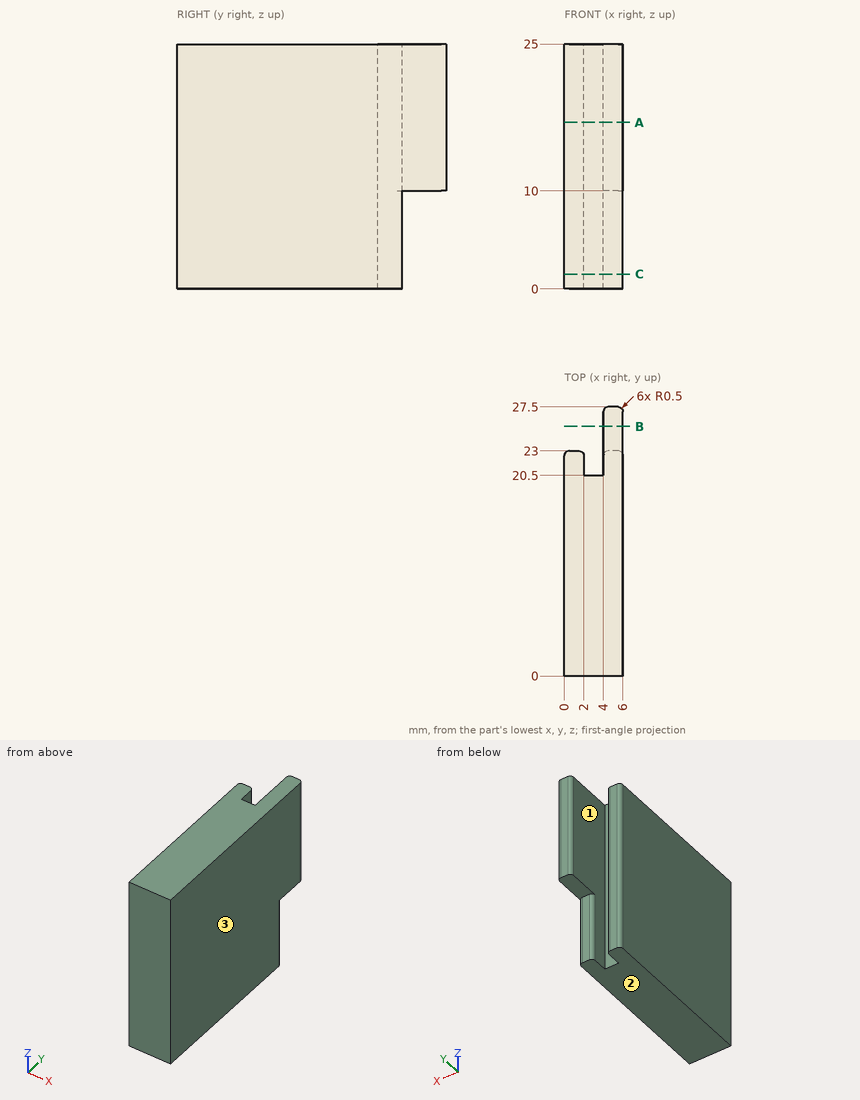
Part print with two shaded views. Sizes in mm from the minimum x, y, z corner. Coordinates: 2 decimals unless noted, no trailing zeros. Write each loop counter-clockwise with the first axis right and the second up, starting at its lowest first coordinate (ties: lowest second). Pieces come first, ordered by that corner, then holes. Notation, with made-up numbers: (37.25, -11) - (83.25, -11) arc R26 ccw to (83.25, 12) - close; hole circle Ø1 at (-20, 6). An arc over 180 degrees is marked (long way). Use a Markdown table: item, result. Add a question column.
Item 1: Two-plate mould, pull along X, no slides. Class the marked faces 1, 2 and 3: pulls with the +X half, pulls with the -X half, needs draft (parallel to the pull), parting line crosses it, or undercut.
Item 2: Drill centre lines: line 1 along X through (y, z) = (22, 16.5); line 2 along Y through (x, z) = (3.6, 21.75); line 3 along Y through (x, z) = (0.6, 4.25). Where is each one in solid material? Low to high.
Item 3: Drop flat-ended pins along their axis: pin 1 (1 mm diameter, centred on x = 1, z = 6.5, fed in from +Y); pin 2 (2 mm diameter, centred on x = 5, y = 25, fed in from -Z); pin 3 (0.6 mm diameter, centred on x = 3, z = 12.5, fed in from +Y). Give the stop position or say it passes through.
Item 4: Band-saw the part on A-A, the plane z = 17. Write the cut outline in (x, y), and give its area (3 significant figures).
Item 5: Band-saw the part on C-C, the plane z = 1.5. Write the cut outline in (x, y), and give its area (3 significant figures).
Item 6: Band-saw the part on B-B, the plane y = 25.5. Write the cut outline in (x, z).
A:
| question | item | result |
|---|---|---|
| 1 | face 1 | undercut |
| 1 | face 2 | needs draft |
| 1 | face 3 | pulls with the +X half |
| 2 | line 1 | x = 0 to 2, 4 to 6 |
| 2 | line 2 | y = 0 to 20.5 |
| 2 | line 3 | y = 0 to 23 |
| 3 | pin 1 | stops at y = 23 |
| 3 | pin 2 | stops at z = 10 |
| 3 | pin 3 | stops at y = 20.5 |
| 4 | outline | (0, 0) - (6, 0) - (6, 27) arc R0.5 ccw to (5.5, 27.5) - (4.5, 27.5) arc R0.5 ccw to (4, 27) - (4, 20.5) - (2, 20.5) - (2, 22.5) arc R0.5 ccw to (1.5, 23) - (0.5, 23) arc R0.5 ccw to (0, 22.5) - close |
| 4 | area | 142 mm² |
| 5 | outline | (0, 0) - (6, 0) - (6, 22.5) arc R0.5 ccw to (5.5, 23) - (4.5, 23) arc R0.5 ccw to (4, 22.5) - (4, 20.5) - (2, 20.5) - (2, 22.5) arc R0.5 ccw to (1.5, 23) - (0.5, 23) arc R0.5 ccw to (0, 22.5) - close |
| 5 | area | 133 mm² |
| 6 | outline | (4, 10) - (6, 10) - (6, 25) - (4, 25) - close |
